```python
from build123d import *

# Parameters (mm, degrees)
CHAMFER_1_SIZE           = 0.2805
SKETCH_4_W               = 1.1
SKETCH_4_H               = 3.2
CUT_EXTRUDE_2_DEPTH      = 3.9
CUT_EXTRUDE_2_DEPTH_BACK = 3.9


with BuildPart() as part:
    # Эскиз1 → Повернуть1 (revolve)
    with BuildSketch(Plane.XY):
        with BuildLine():
            ThreePointArc((0, 2.9), (2.050609665, 2.050609665), (2.9, 0))
            Line((2.9, 0), (1.5, 0))
            Line((1.5, 0), (1.5, -14))
            Line((1.5, -14), (0, -14))
            Line((0, -14), (0, 2.9))
        make_face()
    revolve(axis=Axis((0, 2.9, 0), (0, -1, 0)))

    # Фаска1
    chamfer_1_edges = [part.edges().sort_by_distance(p)[0] for p in [
        (-1.5, -14, 0),
    ]]
    chamfer(chamfer_1_edges, length=CHAMFER_1_SIZE)

    # Эскиз4 → Вырез-Вытянуть2 (cut, two sides)
    with BuildSketch(Plane.XY) as cut_extrude_2_sk:
        with Locations((0, 2.9)):
            Rectangle(SKETCH_4_W, SKETCH_4_H)
    extrude(amount=CUT_EXTRUDE_2_DEPTH, mode=Mode.SUBTRACT)
    extrude(cut_extrude_2_sk.sketch, amount=-CUT_EXTRUDE_2_DEPTH_BACK, mode=Mode.SUBTRACT)


solid = part.part
```
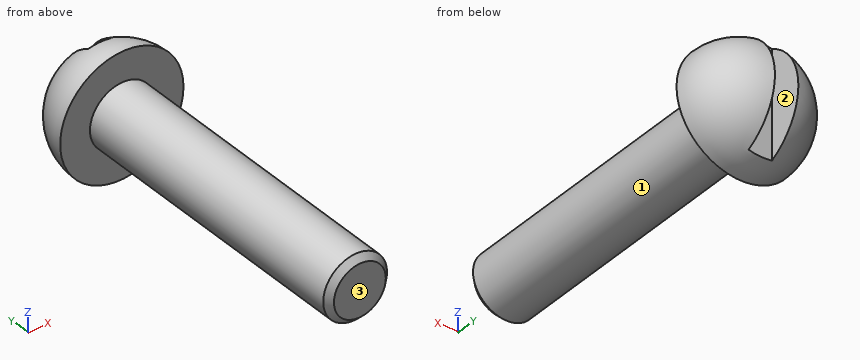
Source: CAD feature listing. Evaluate the final solid. Frame: model axes, mm. Face numbers are marked on the shaded views. A direction names the side the tool comes from. Round coordinates to 2 decimals unless told otherwise and drop trailing zeros. Loops run counter-clockwise (first coordinate to the right, second up) from the corner with the lowest first, then second, coordinate; pieces in that order, holes last. Notation, with made-up numbers: M -4.75,61 L 54.25,61 A19 cw 54.25,66 Z; hole C -1.5,43 d2. An arc over 180 degrees is marked long. Put each result on its own line as item: value.
(1) Section D-D, the plane z = 2.1. Return loops of the section in (x, y), and give its area (3 significant figures).
Solutions:
outline: M -2,0 L 2,0 A2 ccw 0.55,1.92 L 0.55,1.3 L -0.55,1.3 L -0.55,1.92 A2 ccw Z
area: 5.54 mm²
(2) Section C-C, the plane y = -4.25. Return loops of the section in (x, z), and give its area (3 significant figures).
Solutions:
outline: C 0,0 d3
area: 7.07 mm²
(3) Access query for the marked faces 1, 2 and 3. Directions: +Z, -Z, +X, -X, +Y, -Y. A direction counts if a zero-diameter tool reaches every point of the face in a straight line with its end or side. Return the directions, or none.
Solutions:
face 1: -Y
face 2: +Z, -Z, +Y
face 3: +Z, -Z, +X, -X, -Y
(4) First-contact query: pin 1 (3 mm diameter, centred on x = -2, z = 1, fed in from +Y); pin 2 (2 mm diameter, centred on x = 0.5, y = -9.5, fed in from +Z); pin 3 (2 mm diameter, centred on x = 0, y = -10.5, fed in from -Z). Flat tips, straight axial feed; report the tip coordinate or a pass-through.
Solutions:
pin 1: y = 2.81
pin 2: z = 1.5
pin 3: z = -1.5
(5) Section B-B, the plane z = 0. Return loops of the section in (x, y), and give its area (3 significant figures).
Solutions:
outline: M -2.9,0 L -1.5,0 L -1.5,-13.72 L -1.22,-14 L 1.22,-14 L 1.5,-13.72 L 1.5,0 L 2.9,0 A2.9 ccw 0.55,2.85 L 0.55,1.3 L -0.55,1.3 L -0.55,2.85 A2.9 ccw Z
area: 53.4 mm²
(6) Section A-A, the plane x = 0. Return loops of the section in (y, z).
Solutions:
outline: M -14,-1.22 L -13.72,-1.5 L 0,-1.5 L 0,-2.9 A2.9 ccw 1.3,-2.59 L 1.3,2.59 A2.9 ccw 0,2.9 L 0,1.5 L -13.72,1.5 L -14,1.22 Z
(7) Ray query, line 1 (X direction, y = -0.75, z = 0.1); line 2 (X direction, y = 1.5, z = 0.25); line 3 (Y direction, x = -0.9, z = -0.5). Return the intervals inside material, ascending. Write a range as [from, to].
Solutions:
line 1: [-1.5, 1.5]
line 2: [-2.47, -0.55], [0.55, 2.47]
line 3: [-14, 2.71]
